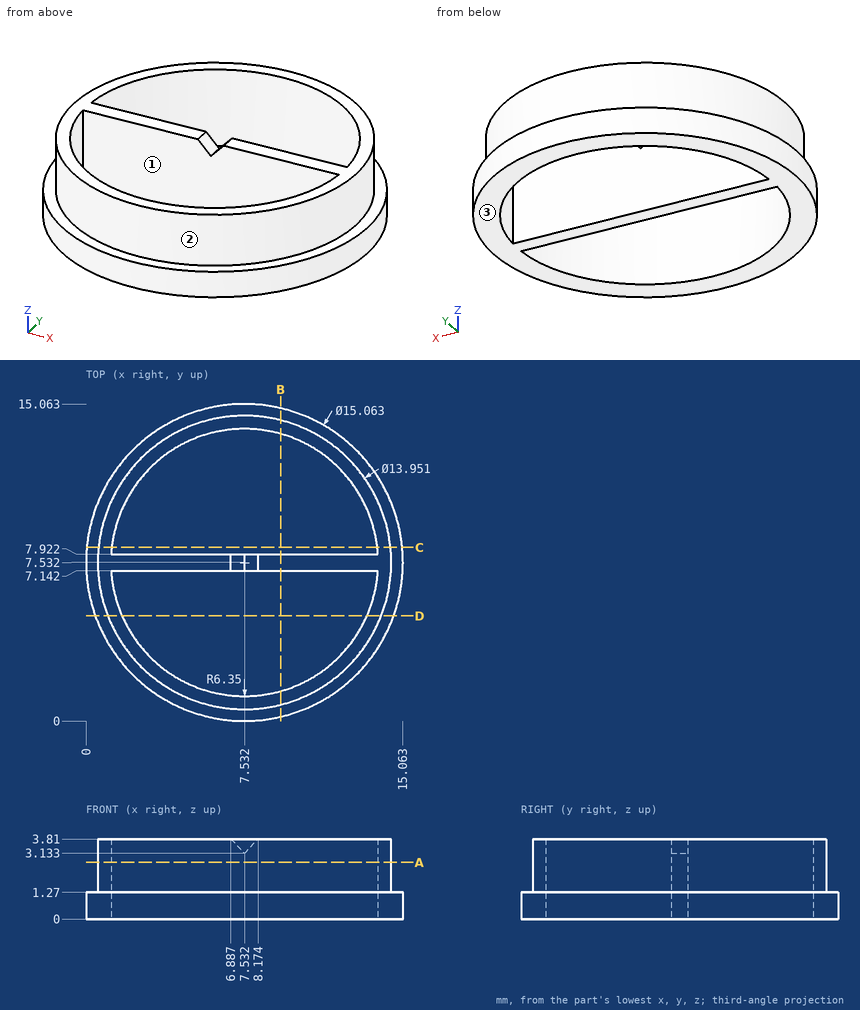
Geometry check sheet. Reference: drawing and pictorial views, mm from the part's lowest x, y, z. Round coordinates to 2 decimals unless told otherwise and drop trailing zeros. Loops run counter-clockwise (first coordinate to the right, second up) from the corner with the lowest first, then second, coordinate; pieces in that order, holes last. Notation, with made-up numbers: (37.25, 3) - (80.25, 3) arc R26 ccw to (80.25, 37) - close; hole circle Ø11 at (-29, 64.5). An arc over 180 degrees is marked (long way). Use a Markdown table: item, result.
Q1. Cross-section at A-A on z = 2.7. State how many separate pieces and enclosed holes the cut face has.
Solutions:
| item | result |
|---|---|
| separate pieces | 1 |
| enclosed holes | 2 |
Q2. Material ranges on line 1 (Y direction, x = 3.25, z = 0.95) (1 decimal); line 2 (Y direction, x = 11.25, z = 0.9) (1 decimal); line 3 (X direction, y = 9.25, z = 3.45) (1 decimal), recorded low to high.
Solutions:
| item | result |
|---|---|
| line 1 | y = 1.3 to 2.8, 7.1 to 7.9, 12.2 to 13.7 |
| line 2 | y = 1 to 2.4, 7.1 to 7.9, 12.7 to 14.1 |
| line 3 | x = 0.8 to 1.4, 13.6 to 14.3 |
Q3. Cross-section at C-C on y = 8.25. Record the cut outline in (x, z) (1 decimal).
Solutions:
| item | result |
|---|---|
| outline | (0, 0) - (1.2, 0) - (1.2, 3.8) - (0.6, 3.8) - (0.6, 1.3) - (0, 1.3) - close; (13.8, 0) - (15, 0) - (15, 1.3) - (14.5, 1.3) - (14.5, 3.8) - (13.8, 3.8) - close |
Q4. Cross-section at B-B on x = 9.25. Record the cut outline in (y, z) (1 decimal).
Solutions:
| item | result |
|---|---|
| outline | (0.2, 0) - (1.4, 0) - (1.4, 3.8) - (0.8, 3.8) - (0.8, 1.3) - (0.2, 1.3) - close; (7.1, 0) - (7.9, 0) - (7.9, 3.8) - (7.1, 3.8) - close; (13.6, 0) - (14.9, 0) - (14.9, 1.3) - (14.3, 1.3) - (14.3, 3.8) - (13.6, 3.8) - close |
Q5. Go/stop test with flat-tipped pins: P1, Ø1.1, axis at x = 5.5, z = 3, coming from the -Y side (1 decimal); P2, Ø1.5, axis at y = 3.5, z = 3, coming from the +X side; P3, Ø1.5, axis at y = 11, z = 1.5, coming from the -X side. Record where each tip stops, or that it passes through.
Solutions:
| item | result |
|---|---|
| P1 | stops at y = 0.7 |
| P2 | stops at x = 13.69 |
| P3 | stops at x = 0.52 |
Q6. Cross-section at D-D on y = 5. Record the cut outline in (x, z) (1 decimal).
Solutions:
| item | result |
|---|---|
| outline | (0.4, 0) - (1.7, 0) - (1.7, 3.8) - (1, 3.8) - (1, 1.3) - (0.4, 1.3) - close; (13.4, 0) - (14.6, 0) - (14.6, 1.3) - (14, 1.3) - (14, 3.8) - (13.4, 3.8) - close |
Q7. Draft check along Y on the marked faces 1, 2 and 3. Enter one of: released by +Y, released by -Y, zero draft, split by the parting line, or undercut.
Solutions:
| item | result |
|---|---|
| face 1 | undercut |
| face 2 | split by the parting line |
| face 3 | zero draft |
